Autodesk Inventor part; units mm, degrees
ref_plane "Work Plane1" through (15.347, 0, 0) normal (0, -1, 0) x (1, 0, 0)
ref_plane "YZ Plane" through (0, 0, 0) normal (1, 0, 0) x (0, 1, 0)
ref_plane "XZ Plane" through (0, 0, 0) normal (0, 1, 0) x (-1, 0, 0)
sketch "Sketch1" plane through (0, 0, 0) normal (1, 0, 0) x (0, 1, 0)
  line L0 (-5.95, 0) -> (5.95, 0)
  line L1 (0, -5.95) -> (0, 5.95)
  line L2 (-5.4, 5.4) -> (5.4, 5.4)
  line L3 (5.4, 5.4) -> (5.4, -5.4)
  line L4 (5.4, -5.4) -> (-5.4, -5.4)
  line L5 (-5.4, -5.4) -> (-5.4, 5.4)
  line L6 (0, 5.4) -> (0, -5.4) construction
  line L7 (-5.4, 0) -> (5.4, 0) construction
  point P0 (0, 0)
  dimension "d0" = 10.8
  dimension "d1" = 10.8
extrude "Body" add sketch "Sketch1" along normal blind 1.5
hole "Hole" at (0, 0, 0) direction (1, 0, 0) diameter 4.05 end through all
ref_plane "Work Plane1" through (15.347, 0, 0) normal (0, -1, 0) x (1, 0, 0)
equation "\"d0\" = SL2"
equation "\"d1\" = SL1"
equation "\"d2\" = SD"
equation "\"d4\" = SD1"
equation "\"SD1\" = 4.05"
equation "\"SL1\" = 10.8"
equation "\"SL2\" = 10.8"
equation "\"SD\" = 1.5"
equation "\"NND\" = 4"
properties part number "IFI - 4" material "Steel, Mild"
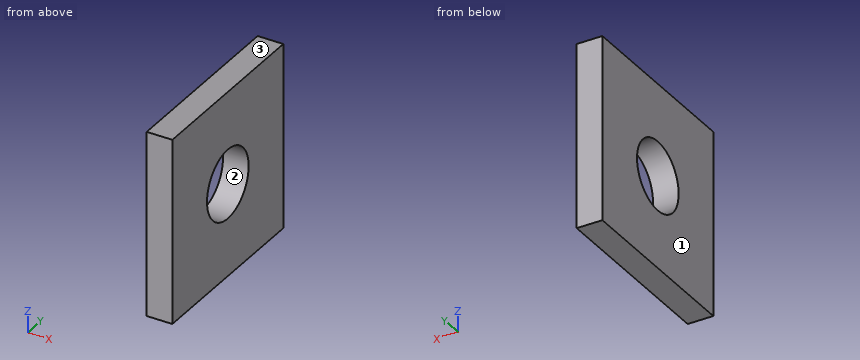
Verification items for the finished model (mm, model axes). Face numbers are marked on the shaded views. Round coordinates to 2 decimals unless told otherwise and drop trailing zeros. Write each loop counter-clockwise with the first axis right and the second up, starting at its lowest first coordinate (ties: lowest second). Pieces come first, ordered by that corner, then holes.
1. Scan line: L1, parallel to Y at x = 0.3, z = 0 (3 decimals). Record every from-to range of solid material in increasing order.
2. Section check A-A on z = 0. Enter the section's corners in (x, y) (3 decimals), plus the area to 3 significant figures.
3. Section check C-C on x = 0.15. Enter the section's corners in (y, z) (3 decimals), plus the area to 3 significant figures.
4. Draft check along Z on the marked faces 1, 2 and 3. Enter one of: +Z half, -Z half, draft (parallel to the pull), parting line (faces both ways), or undercut.
Answer:
1. L1: y = -5.4 to -2.025, 2.025 to 5.4
2. outline: (0, -5.4) - (1.5, -5.4) - (1.5, -2.025) - (0, -2.025) - close; (0, 2.025) - (1.5, 2.025) - (1.5, 5.4) - (0, 5.4) - close
2. area: 10.1 mm2
3. outline: (-5.4, -5.4) - (5.4, -5.4) - (5.4, 5.4) - (-5.4, 5.4) - close; hole circle Ø4.05 at (0, 0)
3. area: 104 mm2
4. face 1: draft
4. face 2: undercut
4. face 3: +Z half
